Model file for the job. Use its own axes, mm. A direction names the side the tool comes from. Coordinates: 2 decimals unless noted, no trailing zeros. Write each loop counter-clockwise with the first axis right and the second up, starting at its lowest first coordinate (ties: lowest second). Pieces come first, ordered by that corner, then holes. Notation, with made-up numbers: (36, 14.25) -> (55, 14.25) arc R28 cw to (55, 52.25) -> close; hole circle Ø10 at (67.5, -34.5). An arc over 180 degrees is marked (long way). Answer as a JSON object with one key per item and string values. Group by question number.
from build123d import *

# Parameters (mm, degrees)
SKETCH1_W           = 56
SKETCH1_H           = 100
BOSS_EXTRUDE1_DEPTH = 55
CUT_EXTRUDE2_DEPTH  = 118.511701545
SKETCH7_R           = 22.5
SKETCH7_R_2         = 10
CUT_EXTRUDE4_DEPTH  = 23
CUT_EXTRUDE5_DEPTH  = 46
CUT_EXTRUDE6_DEPTH  = 3
CUT_EXTRUDE7_DEPTH  = 23
SKETCH12_W          = 15.5
SKETCH12_H          = 17.5
CUT_EXTRUDE8_DEPTH  = 80.429213769
SKETCH13_W          = 25
SKETCH13_H          = 22
CUT_EXTRUDE9_DEPTH  = 118.511701545


with BuildPart() as part:
    # Sketch1 → Boss-Extrude1 (new body)
    with BuildSketch(Plane(origin=(0, 0, 0), x_dir=(1, 0, 0), z_dir=(0, 1, 0))):
        Rectangle(SKETCH1_W, SKETCH1_H)
    extrude(amount=BOSS_EXTRUDE1_DEPTH)

    # Sketch3 → Cut-Extrude2 (cut, through all)
    with BuildSketch(Plane.XY.offset(50)):
        Polygon((-0.5, 32), (-2.5, 55), (2.5, 55), (0.5, 32), align=None)
    extrude(amount=-CUT_EXTRUDE2_DEPTH, mode=Mode.SUBTRACT)

    # Sketch7 → Cut-Extrude4 (cut)
    with BuildSketch(Plane(origin=(0, 55, 0), x_dir=(1, 0, 0), z_dir=(0, 1, 0))):
        with Locations((22, 0)):
            Circle(SKETCH7_R)
        with Locations((22, 0)):
            Circle(SKETCH7_R_2, mode=Mode.SUBTRACT)
    cut_extrude4 = extrude(amount=-CUT_EXTRUDE4_DEPTH, mode=Mode.SUBTRACT)

    # Sketch9 → Cut-Extrude5 (cut)
    with BuildSketch(Plane(origin=(0, 55, 0), x_dir=(1, 0, 0), z_dir=(0, 1, 0))):
        with BuildLine():
            Line((14, 6.408002809), (14, -6.408002809))
            ThreePointArc((14, -6.408002809), (32.25, 0), (14, 6.408002809))
        make_face()
    cut_extrude5 = extrude(amount=-CUT_EXTRUDE5_DEPTH, mode=Mode.SUBTRACT)

    # Sketch10 → Cut-Extrude6 (cut)
    with BuildSketch(Plane(origin=(0, 9, 0), x_dir=(1, 0, 0), z_dir=(0, 1, 0))):
        with BuildLine():
            Line((18, 3), (18, -3))
            ThreePointArc((18, -3), (27, 0), (18, 3))
        make_face()
    cut_extrude6 = extrude(amount=-CUT_EXTRUDE6_DEPTH, mode=Mode.SUBTRACT)

    # Sketch11 → Cut-Extrude7 (cut)
    with BuildSketch(Plane(origin=(0, 55, 0), x_dir=(1, 0, 0), z_dir=(0, 1, 0))):
        with BuildLine():
            Line((14, 6.408002809), (14, -6.408002809))
            ThreePointArc((14, -6.408002809), (11.677076266, 0), (14, 6.408002809))
        make_face()
    cut_extrude7 = extrude(amount=-CUT_EXTRUDE7_DEPTH, mode=Mode.SUBTRACT)

    # Mirror1: Cut-Extrude4, Cut-Extrude5, Cut-Extrude6, Cut-Extrude7 across plane
    add(cut_extrude4.mirror(Plane(origin=(0, 0, 0), x_dir=(0, 0, 1), z_dir=(1, 0, 0))), mode=Mode.SUBTRACT)
    add(cut_extrude5.mirror(Plane(origin=(0, 0, 0), x_dir=(0, 0, 1), z_dir=(1, 0, 0))), mode=Mode.SUBTRACT)
    add(cut_extrude6.mirror(Plane(origin=(0, 0, 0), x_dir=(0, 0, 1), z_dir=(1, 0, 0))), mode=Mode.SUBTRACT)
    add(cut_extrude7.mirror(Plane(origin=(0, 0, 0), x_dir=(0, 0, 1), z_dir=(1, 0, 0))), mode=Mode.SUBTRACT)

    # Sketch12 → Cut-Extrude8 (cut, through all)
    with BuildSketch(Plane(origin=(0, 55, 0), x_dir=(1, 0, 0), z_dir=(0, 1, 0))):
        with Locations((-20.25, 41.25)):
            Rectangle(SKETCH12_W, SKETCH12_H)
        with Locations((20.25, 41.25)):
            Rectangle(SKETCH12_W, SKETCH12_H)
        with Locations((-20.25, -41.25)):
            Rectangle(SKETCH12_W, SKETCH12_H)
        with Locations((20.25, -41.25)):
            Rectangle(SKETCH12_W, SKETCH12_H)
    extrude(amount=-CUT_EXTRUDE8_DEPTH, mode=Mode.SUBTRACT)

    # Sketch13 → Cut-Extrude9 (cut, through all)
    with BuildSketch(Plane.XY.offset(50)):
        with Locations((0, 11)):
            Rectangle(SKETCH13_W, SKETCH13_H)
    extrude(amount=-CUT_EXTRUDE9_DEPTH, mode=Mode.SUBTRACT)


solid = part.part
(1) Cut at A-A on z = 0. List the corners of the cut face in (x, y), plus the area to 3 significant figures.
(2) Cut at D-D on y = 29.5. List the corners of the cut face in (x, z), plus the area to 3 significant figures.
(3) Pin check, flat tips, straight feed: pin 1 (5 mm diameter, centred on y = 36.5, z = -42.5, fed in from +X); pin 2 (11 mm diameter, centred on x = 24.5, z = -5, fed in from +Y); pin 3 (4 mm diameter, centred on y = 10, z = -36, fed in from -X); pin 4 (5 mm diameter, centred on y = 35.5, z = 10.5, fed in from +X). Stop position of each tip, or through.
(4) Wall check: probe 1 along X at (y, z) = (8, 0); probe 2 along Z at (x, y) = (22, 6.85); probe 3 along X at (y, z) = (16, 0). Give the ranges that are in metal, low to high.
(5) Cut at C-C on y = 15.5. List the corners of the cut face in (x, z), plus the area to 3 significant figures.
(6) 3-axis set-ups, long thin cutter, end or side, ignore diameter. For faces 1 (the face through (20, 28, -32.5)), 2 (the face through (10.985, 43.661, 19.619)), 3 (the face through (0, 22, 1)): which of +Z, -Z, +X, -X, +Y, -Y reach the whole face in a straight line?
(7) Cut at B-B on x = -22. List the corners of the cut face in (y, z).
(8) Pull direction Z, two halves, no side cores. Call faces 4 (the face through (17.8, 9, -0.1)), 5 (the face through (-3, 38, -50)), 6 (the face through (-13, 55, -31)), 7 (the face through (-17.8, 9, -0.1)): released by +Z, released by -Z, zero draft, split by the parting line, or undercut.
Results found:
{
 "1": {"outline": "(-28, 0) -> (-12.5, 0) -> (-12.5, 22) -> (12.5, 22) -> (12.5, 0) -> (28, 0) -> (28, 9) -> (27, 9) -> (27, 6) -> (18, 6) -> (18, 9) -> (14, 9) -> (14, 32) -> (-14, 32) -> (-14, 9) -> (-18, 9) -> (-18, 6) -> (-27, 6) -> (-27, 9) -> (-28, 9) -> close", "area": "544 mm²"},
 "2": {"outline": "(-28, -32.5) -> (-12.5, -32.5) -> (-12.5, -50) -> (12.5, -50) -> (12.5, -32.5) -> (28, -32.5) -> (28, -8.31) arc R10.25 cw to (14, -6.41) -> (14, 6.41) arc R10.25 cw to (28, 8.31) -> (28, 32.5) -> (12.5, 32.5) -> (12.5, 50) -> (-12.5, 50) -> (-12.5, 32.5) -> (-28, 32.5) -> (-28, 8.31) arc R10.25 cw to (-14, 6.41) -> (-14, -6.41) arc R10.25 cw to (-28, -8.31) -> close", "area": "3,990 mm²"},
 "3": {"pin 1": "stops at x = 12.5", "pin 2": "stops at y = 32", "pin 3": "passes through", "pin 4": "stops at x = 3.64"},
 "4": {"probe 1": "x = -28 to -27, -18 to -12.5, 12.5 to 18, 27 to 28", "probe 2": "z = -32.5 to -5, 5 to 32.5", "probe 3": "x = -14 to -12.5, 12.5 to 14"},
 "5": {"outline": "(-28, -32.5) -> (-12.5, -32.5) -> (-12.5, 32.5) -> (-28, 32.5) -> (-28, 8.31) arc R10.25 cw to (-14, 6.41) -> (-14, -6.41) arc R10.25 cw to (-28, -8.31) -> close; (12.5, -32.5) -> (28, -32.5) -> (28, -8.31) arc R10.25 cw to (14, -6.41) -> (14, 6.41) arc R10.25 cw to (28, 8.31) -> (28, 32.5) -> (12.5, 32.5) -> close", "area": "1,490 mm²"},
 "6": {"face 1": "-Z, +X, +Y, -Y", "face 2": "+Y", "face 3": "+Z, -Z, -Y"},
 "7": {"outline": "(0, -32.5) -> (55, -32.5) -> (55, -22.5) -> (32, -22.5) -> (32, -10.25) -> (9, -10.25) -> (9, -5) -> (6, -5) -> (6, 5) -> (9, 5) -> (9, 10.25) -> (32, 10.25) -> (32, 22.5) -> (55, 22.5) -> (55, 32.5) -> (0, 32.5) -> close"},
 "8": {"face 4": "undercut", "face 5": "released by -Z", "face 6": "zero draft", "face 7": "undercut"}
}
